Design review of the part built by this model. Coordinates are the model's own, in mm. A direction names the side the tool comes from. Coordinates: 2 decimals unless noted, no trailing zeros. Loops run counter-clockwise (first coordinate to the right, second up) from the corner with the lowest first, then second, coordinate; pieces in that order, holes last. Notation, with made-up numbers: (24.25, 12) - (34.25, 12) arc R20 ccw to (34.25, 34) - close; hole circle Ø3 at (49, 14.25). An arc over 180 degrees is marked (long way). Answer in a Markdown table with one row per item. Add a question column.
(1) Clearance check with flat-ended pins moving along their axes: pin 1 (10 mm diameter, centred on y = -11, z = 61, fed in from -X); pin 2 (4 mm diameter, centred on x = -1, y = -45, fed in from +Z); pin 3 (9 mm diameter, centred on x = 91, y = -36.5, fed in from -Z); pin 4 (3.5 mm diameter, centred on y = -13, z = 190, fed in from +X). State where each tip first meets the part, or that it passes through.
(2) The part is to be moulded in two halves that separate along Z. For faces 1 (the face through (45.561, -71.714, 43.885)), 2 (the face through (90, -26, 207.93)), 3 (the face through (-22.098, -10, 190)), 4 (the face through (152.044, 1.136, 76.898)), say which applies: released by +Z, released by -Z, zero draft, split by the parting line, or undercut.
(3) We need section D-D, the plane z = -21.5. Write out the cut boundary in (x, y), plus the area to 3 significant figures.
(4) We need section C-C, the plane x = 88.9. Write out the cut boundary in (y, z).
(5) To check wall thickness, follow L1, parallel to Y at x = 146, z = 174.5; L2, parallel to Y at x = 88.9, z = 199; L3, parallel to X at y = -35.56, z = 198.5. State the ranges of each line that lie inside material, in increasing order. Write a range as [from, to].
(6) For faces 5 (the face through (1, -7, 193.729)), 6 (the face through (-11, -2.919, 190)), 7 (the face through (0, -10, 162.731)), list the 3-axis set-ups (+Z, -Z, +X, -X, +Y, -Y) from which the entire face can be reached by the end or side of a thin tool; tool diameter is ignored.
(7) We need section A-A, the plane x = 63.5. Write out the cut boundary in (y, z), plus the area to 3 significant figures.
(8) We need section B-B, the plane y = -35.56. Write out the cut boundary in (x, z).
from build123d import *

# Parameters (mm, degrees)
SALIENTE_EXTRUIR1_DEPTH       = 4.572
CROQUIS2_W                    = 4.572
CROQUIS2_H                    = 76.2
SALIENTE_EXTRUIR2_DEPTH       = 177.8
SALIENTE_EXTRUIR3_DEPTH       = 5.08
SALIENTE_EXTRUIR3_DEPTH_BACK  = 76.2
CORTAR_EXTRUIR5_DEPTH         = 208.534
CROQUIS5_R                    = 12.7
CORTAR_EXTRUIR6_DEPTH         = 50.038
CORTAR_EXTRUIR6_DEPTH_BACK    = 148.336
CROQUIS6_R                    = 22.606
CORTAR_EXTRUIR12_DEPTH        = 33.274
CORTAR_EXTRUIR12_DEPTH_BACK   = 97.282
CROQUIS7_R                    = 7.975525782
CORTAR_EXTRUIR13_DEPTH        = 66.04
CORTAR_EXTRUIR13_DEPTH_BACK   = 177.8
CROQUIS8_R                    = 8.001
CROQUIS8_R_2                  = 7.975525782
SALIENTE_EXTRUIR8_DEPTH       = 19.304
SALIENTE_EXTRUIR8_DEPTH_BACK  = 18.034
CROQUIS9_R                    = 8.001
SALIENTE_EXTRUIR9_DEPTH       = 15.494
SALIENTE_EXTRUIR9_DEPTH_BACK  = 19.558
CROQUIS10_W                   = 16.002
CROQUIS10_H                   = 15.494
CORTAR_EXTRUIR14_DEPTH        = 261.874
CORTAR_EXTRUIR15_DEPTH        = 422.402
CROQUIS12_R                   = 8.001
SALIENTE_EXTRUIR10_DEPTH      = 118.618
CROQUIS13_W                   = 16.002
CROQUIS13_H                   = 64.433284084
CORTAR_EXTRUIR16_DEPTH        = 300.99
CORTAR_EXTRUIR17_DEPTH        = 262.89
CROQUIS15_R                   = 3.175
CORTAR_EXTRUIR18_DEPTH        = 120.142
CORTAR_EXTRUIR18_DEPTH_BACK   = 292.1
CROQUIS16_R                   = 4.7625
CORTAR_EXTRUIR20_DEPTH        = 446.532
CROQUIS20_R                   = 9.023236634
CROQUIS20_R_2                 = 5.413941981
SALIENTE_EXTRUIR12_DEPTH      = 206.502
SALIENTE_EXTRUIR12_DEPTH_BACK = 2.54
CROQUIS22_W                   = 184.818676859
CROQUIS22_H                   = 18.046473268
CORTAR_EXTRUIR21_DEPTH        = 252.984
CROQUIS23_W                   = 10.680092276
CROQUIS23_H                   = 18.046473268
CORTAR_EXTRUIR22_DEPTH        = 336.55
CROQUIS24_W                   = 7.23294038
CROQUIS24_H                   = 8.186318229
SALIENTE_EXTRUIR13_DEPTH      = 23.876
SALIENTE_EXTRUIR13_DEPTH_BACK = 22.098
CROQUIS25_W                   = 45.974
CROQUIS25_H                   = 6.021939504
SALIENTE_EXTRUIR14_DEPTH      = 193.548
SALIENTE_EXTRUIR14_DEPTH_BACK = 5.08
CROQUIS26_W                   = 191.576169951
CROQUIS26_H                   = 6.021939504
CORTAR_EXTRUIR23_DEPTH        = 184.658
CORTAR_EXTRUIR23_DEPTH_BACK   = 81.534
CROQUIS27_W                   = 8.610643309
CROQUIS27_H                   = 14.208257733
SALIENTE_EXTRUIR15_DEPTH      = 22.86
SALIENTE_EXTRUIR15_DEPTH_BACK = 23.622
CROQUIS28_R                   = 3.97256
CORTAR_EXTRUIR24_DEPTH        = 207.01


with BuildPart() as part:
    # Croquis1 → Saliente-Extruir1 (new body)
    with BuildSketch(Plane(origin=(0, 0, 0), x_dir=(1, 0, 0), z_dir=(0, 1, 0))):
        Polygon((0, 46.07031702), (0, -207.92968298), (177.8, -207.92968298), (127, 46.07031702), align=None)
    extrude(amount=SALIENTE_EXTRUIR1_DEPTH)

    # Croquis2 → Saliente-Extruir2 (add)
    with BuildSketch(Plane(origin=(0, 0, 0), x_dir=(0, 0, -1), z_dir=(1, 0, 0))):
        with Locations((-205.64368298, -33.528)):
            Rectangle(CROQUIS2_W, CROQUIS2_H)
    extrude(amount=SALIENTE_EXTRUIR2_DEPTH)

    # Croquis3 → Saliente-Extruir3 (add, two sides)
    with BuildSketch(Plane(origin=(0, 0, 0), x_dir=(1, 0, 0), z_dir=(0, 1, 0))) as saliente_extruir3_sk:
        Polygon((0, -207.92968298), (0, 46.07031702), (127, 46.07031702), (177.8, -203.35768298), (177.8, -207.92968298), align=None)
    extrude(amount=SALIENTE_EXTRUIR3_DEPTH)
    extrude(saliente_extruir3_sk.sketch, amount=-SALIENTE_EXTRUIR3_DEPTH_BACK)

    # Croquis4 → Cortar-Extruir5 (cut)
    with BuildSketch(Plane(origin=(0, 0, 0), x_dir=(0, 0, -1), z_dir=(1, 0, 0))):
        Polygon((46.07031702, -2.919454773), (46.07031702, -67.352738857), (-203.792527081, -67.352738857), (-203.35768298, -2.919454773), align=None)
    extrude(amount=CORTAR_EXTRUIR5_DEPTH, mode=Mode.SUBTRACT)

    # Croquis5 → Cortar-Extruir6 (cut, two sides)
    with BuildSketch(Plane(origin=(0, 0, 0), x_dir=(1, 0, 0), z_dir=(0, 1, 0))) as cortar_extruir6_sk:
        with Locations((63.5, -30.12968298)):
            Circle(CROQUIS5_R)
    extrude(amount=CORTAR_EXTRUIR6_DEPTH, mode=Mode.SUBTRACT)
    extrude(cortar_extruir6_sk.sketch, amount=-CORTAR_EXTRUIR6_DEPTH_BACK, mode=Mode.SUBTRACT)

    # Croquis6 → Cortar-Extruir12 (cut, two sides)
    with BuildSketch(Plane(origin=(0, 0, 0), x_dir=(1, 0, 0), z_dir=(0, 1, 0))) as cortar_extruir12_sk:
        with Locations((63.5, -30.12968298)):
            Circle(CROQUIS6_R)
    extrude(amount=CORTAR_EXTRUIR12_DEPTH, mode=Mode.SUBTRACT)
    extrude(cortar_extruir12_sk.sketch, amount=-CORTAR_EXTRUIR12_DEPTH_BACK, mode=Mode.SUBTRACT)

    # Croquis7 → Cortar-Extruir13 (cut, two sides)
    with BuildSketch(Plane(origin=(0, 0, 0), x_dir=(1, 0, 0), z_dir=(0, 1, 0))) as cortar_extruir13_sk:
        with Locations((122.352899809, -133.656770096)):
            Circle(CROQUIS7_R)
    extrude(amount=CORTAR_EXTRUIR13_DEPTH, mode=Mode.SUBTRACT)
    extrude(cortar_extruir13_sk.sketch, amount=-CORTAR_EXTRUIR13_DEPTH_BACK, mode=Mode.SUBTRACT)

    # Croquis8 → Saliente-Extruir8 (add, two sides)
    with BuildSketch(Plane.XZ.offset(76.2)) as saliente_extruir8_sk:
        with Locations((122.352899809, 133.656770096)):
            Circle(CROQUIS8_R)
        with Locations((122.352899809, 133.656770096)):
            Circle(CROQUIS8_R_2, mode=Mode.SUBTRACT)
    extrude(amount=SALIENTE_EXTRUIR8_DEPTH)
    extrude(saliente_extruir8_sk.sketch, amount=-SALIENTE_EXTRUIR8_DEPTH_BACK)

    # Croquis9 → Saliente-Extruir9 (add, two sides)
    with BuildSketch(Plane(origin=(0, 5.08, 0), x_dir=(1, 0, 0), z_dir=(0, 1, 0))) as saliente_extruir9_sk:
        with Locations((122.352899809, -133.656770096)):
            Circle(CROQUIS9_R)
    extrude(amount=SALIENTE_EXTRUIR9_DEPTH)
    extrude(saliente_extruir9_sk.sketch, amount=-SALIENTE_EXTRUIR9_DEPTH_BACK)

    # Croquis10 → Cortar-Extruir14 (cut)
    with BuildSketch(Plane(origin=(0, 0, 0), x_dir=(0, 0, -1), z_dir=(1, 0, 0))):
        with Locations((-133.656770096, 12.827)):
            Rectangle(CROQUIS10_W, CROQUIS10_H)
    extrude(amount=CORTAR_EXTRUIR14_DEPTH, mode=Mode.SUBTRACT)

    # Croquis11 → Cortar-Extruir15 (cut)
    with BuildSketch(Plane(origin=(0, 0, 0), x_dir=(0, 0, -1), z_dir=(1, 0, 0))):
        Polygon((-142.139346511, -2.919454773), (-142.052853493, -14.491925991), (-125.655770096, -14.478), (-125.655770096, -2.919454773), align=None)
        Polygon((-141.657770096, -67.352738857), (-125.655770096, -67.352738857), (-125.655770096, -57.997233167), (-141.727693443, -57.997233167), align=None)
    extrude(amount=CORTAR_EXTRUIR15_DEPTH, mode=Mode.SUBTRACT)

    # Croquis12 → Saliente-Extruir10 (add)
    with BuildSketch(Plane(origin=(0, 0, 0), x_dir=(1, 0, 0), z_dir=(0, 1, 0))):
        with Locations((122.352899809, -133.656770096)):
            Circle(CROQUIS12_R)
    extrude(amount=-SALIENTE_EXTRUIR10_DEPTH)

    # Croquis13 → Cortar-Extruir16 (cut)
    with BuildSketch(Plane(origin=(0, 0, 0), x_dir=(0, 0, -1), z_dir=(1, 0, 0))):
        with Locations((-133.656770096, -35.136096815)):
            Rectangle(CROQUIS13_W, CROQUIS13_H)
    extrude(amount=CORTAR_EXTRUIR16_DEPTH, mode=Mode.SUBTRACT)

    # Croquis14 → Cortar-Extruir17 (cut)
    with BuildSketch(Plane(origin=(0, 0, 0), x_dir=(0, 0, -1), z_dir=(1, 0, 0))):
        Polygon((-141.823129416, -76.2), (-141.657770096, -118.618), (-125.655770096, -118.618), (-125.655770096, -76.2), align=None)
    extrude(amount=CORTAR_EXTRUIR17_DEPTH, mode=Mode.SUBTRACT)

    # Croquis15 → Cortar-Extruir18 (cut, two sides)
    with BuildSketch(Plane(origin=(0, 0, 0), x_dir=(1, 0, 0), z_dir=(0, 1, 0))) as cortar_extruir18_sk:
        with Locations((126.414802626, -142.640423395)):
            Circle(CROQUIS15_R)
    extrude(amount=CORTAR_EXTRUIR18_DEPTH, mode=Mode.SUBTRACT)
    extrude(cortar_extruir18_sk.sketch, amount=-CORTAR_EXTRUIR18_DEPTH_BACK, mode=Mode.SUBTRACT)

    # Croquis16 → Cortar-Extruir20 (cut)
    with BuildSketch(Plane.XY):
        with Locations((88.9, -35.56)):
            Circle(CROQUIS16_R)
    extrude(amount=CORTAR_EXTRUIR20_DEPTH, mode=Mode.SUBTRACT)

    # Croquis20 → Saliente-Extruir12 (add, two sides)
    with BuildSketch(Plane.XY) as saliente_extruir12_sk:
        with Locations((88.9, -35.56)):
            Circle(CROQUIS20_R)
        with Locations((88.9, -35.56)):
            Circle(CROQUIS20_R_2, mode=Mode.SUBTRACT)
    extrude(amount=SALIENTE_EXTRUIR12_DEPTH)
    extrude(saliente_extruir12_sk.sketch, amount=-SALIENTE_EXTRUIR12_DEPTH_BACK)

    # Croquis22 → Cortar-Extruir21 (cut)
    with BuildSketch(Plane(origin=(0, 0, 0), x_dir=(0, 0, -1), z_dir=(1, 0, 0))):
        with Locations((-89.86933843, -35.56)):
            Rectangle(CROQUIS22_W, CROQUIS22_H)
    extrude(amount=CORTAR_EXTRUIR21_DEPTH, mode=Mode.SUBTRACT)

    # Croquis23 → Cortar-Extruir22 (cut)
    with BuildSketch(Plane(origin=(0, 0, 0), x_dir=(0, 0, -1), z_dir=(1, 0, 0))):
        with Locations((-187.618722997, -35.56)):
            Rectangle(CROQUIS23_W, CROQUIS23_H)
    extrude(amount=CORTAR_EXTRUIR22_DEPTH, mode=Mode.SUBTRACT)

    # Croquis24 → Saliente-Extruir13 (add, two sides)
    with BuildSketch(Plane(origin=(0, 0, 0), x_dir=(0, 0, -1), z_dir=(1, 0, 0))) as saliente_extruir13_sk:
        with Locations((-190.112640141, -7.012613888)):
            Rectangle(CROQUIS24_W, CROQUIS24_H)
    extrude(amount=SALIENTE_EXTRUIR13_DEPTH)
    extrude(saliente_extruir13_sk.sketch, amount=-SALIENTE_EXTRUIR13_DEPTH_BACK)

    # Croquis25 → Saliente-Extruir14 (add, two sides)
    with BuildSketch(Plane.XY) as saliente_extruir14_sk:
        with Locations((0.889, -14.116742754)):
            Rectangle(CROQUIS25_W, CROQUIS25_H)
    extrude(amount=SALIENTE_EXTRUIR14_DEPTH)
    extrude(saliente_extruir14_sk.sketch, amount=-SALIENTE_EXTRUIR14_DEPTH_BACK)

    # Croquis26 → Cortar-Extruir23 (cut, two sides)
    with BuildSketch(Plane(origin=(0, 0, 0), x_dir=(0, 0, -1), z_dir=(1, 0, 0))) as cortar_extruir23_sk:
        with Locations((-90.708084976, -14.116742754)):
            Rectangle(CROQUIS26_W, CROQUIS26_H)
    extrude(amount=CORTAR_EXTRUIR23_DEPTH, mode=Mode.SUBTRACT)
    extrude(cortar_extruir23_sk.sketch, amount=-CORTAR_EXTRUIR23_DEPTH_BACK, mode=Mode.SUBTRACT)

    # Croquis27 → Saliente-Extruir15 (add, two sides)
    with BuildSketch(Plane(origin=(0, 0, 0), x_dir=(0, 0, -1), z_dir=(1, 0, 0))) as saliente_extruir15_sk:
        with Locations((-167.036116073, -10.023583639)):
            Rectangle(CROQUIS27_W, CROQUIS27_H)
    extrude(amount=SALIENTE_EXTRUIR15_DEPTH)
    extrude(saliente_extruir15_sk.sketch, amount=-SALIENTE_EXTRUIR15_DEPTH_BACK)

    # Croquis28 → Cortar-Extruir24 (cut)
    with BuildSketch(Plane.XY):
        with Locations((-15.911630765, -10.02358364)):
            Circle(CROQUIS28_R)
    extrude(amount=CORTAR_EXTRUIR24_DEPTH, mode=Mode.SUBTRACT)


solid = part.part
Responses:
| question | item | result |
|---|---|---|
| 1 | pin 1 | passes through |
| 1 | pin 2 | stops at z = 207.93 |
| 1 | pin 3 | stops at z = 192.96 |
| 1 | pin 4 | stops at x = 23.88 |
| 2 | face 1 | undercut |
| 2 | face 2 | released by +Z |
| 2 | face 3 | zero draft |
| 2 | face 4 | released by -Z |
| 3 | outline | (0, -76.2) - (132, -76.2) - (132, -67.35) - (0, -67.35) - close; (0, -2.92) - (132, -2.92) - (132, 5.08) - (0, 5.08) - close |
| 3 | area | 2,220 mm2 |
| 4 | outline | (-76.2, -46.07) - (-67.35, -46.07) - (-67.35, 203.79) - (-44.58, 203.64) - (-44.58, 192.96) - (-40.97, 192.96) - (-40.97, 203.61) - (-40.32, 203.61) - (-40.32, 207.93) - (-76.2, 207.93) - close; (-30.8, 203.55) - (-30.15, 203.54) - (-30.15, 192.96) - (-26.54, 192.96) - (-26.54, 203.52) - (-2.92, 203.36) - (-2.92, -46.07) - (5.08, -46.07) - (5.08, 207.93) - (-30.8, 207.93) - close |
| 5 | L1 | y = [-76.2, -67.35], [-2.92, 5.08] |
| 5 | L2 | y = [-76.2, -67.35], [-44.58, -40.97], [-30.15, -26.54], [-2.92, 5.08] |
| 5 | L3 | x = [79.88, 83.49], [94.31, 97.92] |
| 6 | face 5 | +X, -X |
| 6 | face 6 | +Z, -Z, -X, +Y |
| 6 | face 7 | -Z, +X, -X |
| 7 | outline | (-76.2, -46.07) - (-67.35, -46.07) - (-67.35, 7.52) - (-76.2, 7.52) - close; (-76.2, 52.74) - (-67.35, 52.74) - (-67.35, 203.79) - (-2.92, 203.36) - (-2.92, 52.74) - (5.08, 52.74) - (5.08, 207.93) - (-76.2, 207.93) - close; (-2.92, -46.07) - (5.08, -46.07) - (5.08, 7.52) - (-2.92, 7.52) - close |
| 7 | area | 3,800 mm2 |
| 8 | outline | (0, 203.58) - (79.88, 203.58) - (79.88, 192.96) - (83.49, 192.96) - (83.49, 203.58) - (84.14, 203.58) - (84.14, 207.93) - (0, 207.93) - close; (93.66, 203.58) - (94.31, 203.58) - (94.31, 192.96) - (97.92, 192.96) - (97.92, 203.58) - (177.8, 203.58) - (177.8, 207.93) - (93.66, 207.93) - close |
